```python
from build123d import *

# Parameters (mm, degrees)
F0_W     = 69.85
F0_H     = 44.45
F1_DEPTH = 25.4
F2_W     = 25.4
F2_H     = 25.4
F3_DEPTH = 25.4
F5_DEPTH = 25.4
F7_DEPTH = 25.4
F9_DEPTH = 44.451


with BuildPart() as f1:
    # F0 (on Front) → F1 (new body)
    with BuildSketch(Plane.XZ):
        with Locations((34.925, 22.225)):
            Rectangle(F0_W, F0_H)
    extrude(amount=F1_DEPTH)

    # F2 (on face) → F3 (cut)
    with BuildSketch(Plane.XY.offset(44.45)):
        with Locations((12.7, -12.7)):
            Rectangle(F2_W, F2_H)
        with Locations((57.15, -12.7)):
            Rectangle(F2_W, F2_H)
    extrude(amount=-F3_DEPTH, mode=Mode.SUBTRACT)

    # F4 (on face) → F5 (cut)
    with BuildSketch(Plane.XY.offset(19.05)):
        with BuildLine():
            ThreePointArc((19.1716522932, -12.7), (17.276149222, -8.123850778), (12.7, -6.2283477068))
            Line((12.7, -6.2283477068), (12.7, -19.1716522932))
            ThreePointArc((12.7, -19.1716522932), (17.276149222, -17.276149222), (19.1716522932, -12.7))
        make_face()
        with BuildLine():
            Line((12.7, -19.1716522932), (12.7, -6.2283477068))
            ThreePointArc((12.7, -6.2283477068), (6.2283477068, -12.7), (12.7, -19.1716522932))
        make_face()
        with BuildLine():
            ThreePointArc((0, -9.8877794327), (4.3409961707, -2.8703305999), (12.0772768095, 0))
            Line((12.0772768095, 0), (0, 0))
            Line((0, 0), (0, -9.8877794327))
        make_face()
        with BuildLine():
            ThreePointArc((12.0772768095, -25.4), (4.3409961707, -22.5296694001), (0, -15.5122205673))
            Line((0, -15.5122205673), (0, -25.4))
            Line((0, -25.4), (12.0772768095, -25.4))
        make_face()
    extrude(amount=-F5_DEPTH, mode=Mode.SUBTRACT)

    # F6 (on face) → F7 (cut)
    with BuildSketch(Plane.XY.offset(19.05)):
        with BuildLine():
            Line((57.15, -19.2128030993), (57.15, -6.1871969007))
            ThreePointArc((57.15, -6.1871969007), (50.6371969007, -12.7), (57.15, -19.2128030993))
        make_face()
        with BuildLine():
            ThreePointArc((63.6628030993, -12.7), (61.7552472361, -8.0947527639), (57.15, -6.1871969007))
            Line((57.15, -6.1871969007), (57.15, -19.2128030993))
            ThreePointArc((57.15, -19.2128030993), (61.7552472361, -17.3052472361), (63.6628030993, -12.7))
        make_face()
        with BuildLine():
            Line((69.85, 0), (57.6164578164, 0))
            ThreePointArc((57.6164578164, 0), (65.5484324783, -2.9699513679), (69.85, -10.2660702007))
            Line((69.85, -10.2660702007), (69.85, 0))
        make_face()
        with BuildLine():
            Line((69.85, -25.4), (69.85, -15.1339297993))
            ThreePointArc((69.85, -15.1339297993), (65.5484324783, -22.4300486321), (57.6164578164, -25.4))
            Line((57.6164578164, -25.4), (69.85, -25.4))
        make_face()
    extrude(amount=-F7_DEPTH, mode=Mode.SUBTRACT)

    # F8 (on face) → F9 (cut, through all)
    with BuildSketch(Plane.YZ.offset(44.45)):
        with BuildLine():
            Line((-19.156636307, 31.75), (-6.243363693, 31.75))
            ThreePointArc((-6.243363693, 31.75), (-12.7, 38.206636307), (-19.156636307, 31.75))
        make_face()
        with BuildLine():
            ThreePointArc((-19.156636307, 31.75), (-12.7, 25.293363693), (-6.243363693, 31.75))
            Line((-6.243363693, 31.75), (-19.156636307, 31.75))
        make_face()
        with BuildLine():
            ThreePointArc((-25.4, 31.75), (-12.7, 44.1159367091), (0, 31.75))
            Line((0, 31.75), (0, 44.45))
            Line((0, 44.45), (-25.4, 44.45))
            Line((-25.4, 44.45), (-25.4, 31.75))
        make_face()
    extrude(amount=-F9_DEPTH, mode=Mode.SUBTRACT)


solid = f1.part
```
Could you check a few things on this model? Use its own coordinates, in mm. A direction names the side the tool comes from. Round coordinates to 2 decimals unless told otherwise and drop trailing zeros. Order: outer loops, then holes, each group sorted by start corner. A loop starts at its lowest first (then second) coordinate and runs counter-clockwise, first axis right, second up. Notation, with made-up numbers: (41.25, 40.5) -> (69.25, 40.5) arc R23 ccw to (69.25, 55.5) -> close; hole circle Ø8 at (77.25, -12). An arc over 180 degrees is marked (long way). One line per question, with ' | ' between items.
Q1. If we section it at C-C on z = 27.5: Write out the boundary of the cut face in (x, y).
Computed values:
outline: (25.4, -25.4) -> (44.45, -25.4) -> (44.45, -17.56) -> (25.4, -17.56) -> close; (25.4, -7.84) -> (44.45, -7.84) -> (44.45, 0) -> (25.4, 0) -> close
Q2. Which directions (+Z, -Z, +X, -X, +Y, -Y) give clear straight access to the entire face, cutting with the end or side of a thin tool? Please do faces 1 (the face through (51, -10, 19.05)), 2 (the face through (35, 0, 13)), 3 (the face through (25.4, -13, 23)).
Computed values:
face 1: +Z, +X, +Y, -Y | face 2: +Z, -Z, +X, -X, +Y | face 3: +Z, -X, +Y, -Y
Q3. If we section it at B-B on z = 4: Write out the boundary of the cut face in (x, y).
Computed values:
outline: (0, -15.51) arc R12.7 ccw to (12.08, -25.4) -> (57.62, -25.4) arc R12.7 ccw to (69.85, -15.13) -> (69.85, -10.27) arc R12.7 ccw to (57.62, 0) -> (12.08, 0) arc R12.7 ccw to (0, -9.89) -> close; hole circle Ø12.94 at (12.7, -12.7); hole circle Ø13.03 at (57.15, -12.7)
Q4. If we section it at A-A on x = 58.5: Write out the boundary of the cut face in (y, z).
Computed values:
outline: (-25.35, 0) -> (-19.07, 0) -> (-19.07, 19.05) -> (-25.35, 19.05) -> close; (-6.33, 0) -> (-0.05, 0) -> (-0.05, 19.05) -> (-6.33, 19.05) -> close
Q5. I'm going to push flat-ended pins straight in: pin 1 (12 mm diameter, centred on x = 12.5, y = -6.5, fed in from +Z); pin 2 (12.5 mm diameter, centred on y = -16, z = 31, fed in from -X). Where does each tip first touch, or does it pass through?
Computed values:
pin 1: z = 19.05 | pin 2: x = 25.4
Q6. If I drill on line 1 (Z direction, x = 33.5, y = -12.7); line 2 (Y direction, x = 29.5, z = 31.75); line 3 (X direction, y = -10.5, z = 11), over which ranges is the centre line in solid material (lowest first)? Write a range as from..to.
Computed values:
line 1: 0..25.29, 38.21..44.12 | line 2: -25.4..-19.16, -6.24..0 | line 3: 0..6.61, 18.79..51.02, 63.28..69.85
